```python
from build123d import *

# Parameters (mm, degrees)
BOSS_EXTRUDE1_DEPTH   = 0.4064
F_4_CLEARANCE_HOLE1_D = 3.2639
SKETCH5_R             = 6.35
CUT_EXTRUDE1_DEPTH    = 0.4064


with BuildPart() as part:
    # Sketch1 → Boss-Extrude1 (new body)
    with BuildSketch(Plane.XY):
        Polygon((22.499532885, 9.7155), (27.0002, 5.214832885), (27.0002, -5.214832885), (22.499532885, -9.7155), (-22.499532885, -9.7155), (-27.0002, -5.214832885), (-27.0002, 5.214832885), (-22.499532885, 9.7155), align=None)
    extrude(amount=BOSS_EXTRUDE1_DEPTH)

    # #4 Clearance Hole1 (through all)
    with Locations(Plane.XY.offset(0.4064)):
        with Locations((-23.241, 0), (23.241, 0)):
            Hole(F_4_CLEARANCE_HOLE1_D / 2)

    # Sketch5 → Cut-Extrude1 (cut)
    with BuildSketch(Plane.XY.offset(0.4064)):
        Circle(SKETCH5_R)
    extrude(amount=-CUT_EXTRUDE1_DEPTH, mode=Mode.SUBTRACT)


solid = part.part
```
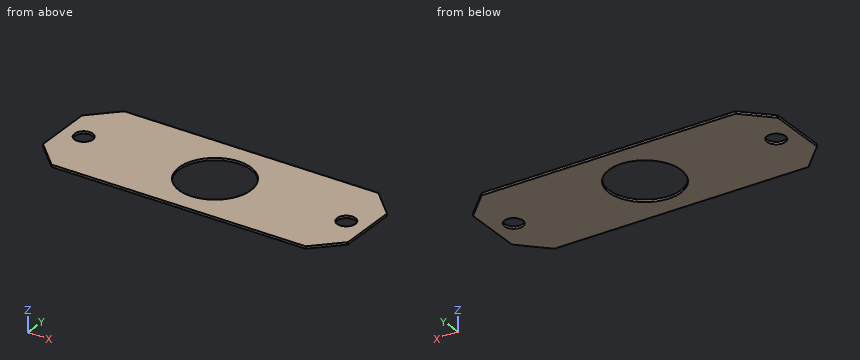
The model under review builds one solid part; all positions refer to its coordinate system, in mm. Round coordinates to 2 decimals unless told otherwise and drop trailing zeros. Write each loop counter-clockwise with the first axis right and the second up, starting at its lowest first coordinate (ties: lowest second). Pieces come first, ordered by that corner, then holes.
(1) We need section D-D on y = -4.75. Give the boundary of the cut face in (x, z).
(2) We need section B-B on y = 0. Give the boundary of the cut face in (x, z).
(3) Wall thickness on L1, parallel to Y at x = 0, z = 0.3; L2, parallel to X at y = 1.25, z = 0.2; L3, parallel to X at y = 0.75, z = 0.35: over which ranges is each line inside the solid? List them lowest first.
(4) We need section C-C on z = 0.15. Give the boundary of the cut face in (x, y).
(5) We need section A-A on x = 0. Give the boundary of the cut face in (y, z).
Findings below:
1. outline: (-27, 0) - (-4.21, 0) - (-4.21, 0.41) - (-27, 0.41) - close; (4.21, 0) - (27, 0) - (27, 0.41) - (4.21, 0.41) - close
2. outline: (-27, 0) - (-24.87, 0) - (-24.87, 0.41) - (-27, 0.41) - close; (-21.61, 0) - (-6.35, 0) - (-6.35, 0.41) - (-21.61, 0.41) - close; (6.35, 0) - (21.61, 0) - (21.61, 0.41) - (6.35, 0.41) - close; (24.87, 0) - (27, 0) - (27, 0.41) - (24.87, 0.41) - close
3. L1: y = -9.72 to -6.35, 6.35 to 9.72
3. L2: x = -27 to -24.29, -22.19 to -6.23, 6.23 to 22.19, 24.29 to 27
3. L3: x = -27 to -24.69, -21.79 to -6.31, 6.31 to 21.79, 24.69 to 27
4. outline: (-27, -5.21) - (-22.5, -9.72) - (22.5, -9.72) - (27, -5.21) - (27, 5.21) - (22.5, 9.72) - (-22.5, 9.72) - (-27, 5.21) - close; hole circle Ø3.26 at (-23.24, 0); hole circle Ø12.7 at (0, 0); hole circle Ø3.26 at (23.24, 0)
5. outline: (-9.72, 0) - (-6.35, 0) - (-6.35, 0.41) - (-9.72, 0.41) - close; (6.35, 0) - (9.72, 0) - (9.72, 0.41) - (6.35, 0.41) - close
